Job drawing, mm, ordinate dimensions from the low corner. One solid piece. A direction names the side the tool comes from. Round coordinates to 2 decimals unless told otherwise and drop trailing zeros. Loops run counter-clockwise (first coordinate to the right, second up) from the corner with the lowest first, then second, coordinate; pieces in that order, holes last.
1) 3-axis set-ups, long thin cutter, end or side, ignore diameter. For the marked faces 1 and 2: which of +Z, -Z, +X, -X, +Y, -Y reach the whole face in a straight line?
2) Band-saw the part on B-B, the plane x = 48.5. Write the cut outline in (y, z).
3) Mould opens along Z. For the marked faces 3, 4 and 5 say: +Z half, -Z half, draft (parallel to the pull), parting line (faces both ways), or undercut.
4) Probe line 1 (X direction, y = 16, z = 61); line 2 (Z direction, x = 138.5, y = 27). List the from-to ranges inside material, lowest first.
5) Drop a flat-ended pin along its axis: P1, Ø10, axis at x = 246.5, y = 14.5, coming from the -Z side. Give the stop position or say it passes through.
6) Band-saw the part on C-C, the plane z = 81.5. Write the cut outline in (x, y).
7) Band-saw the part on A-A, the plane y = 23. Write the cut outline in (x, z), then the cut area to 3 significant figures.
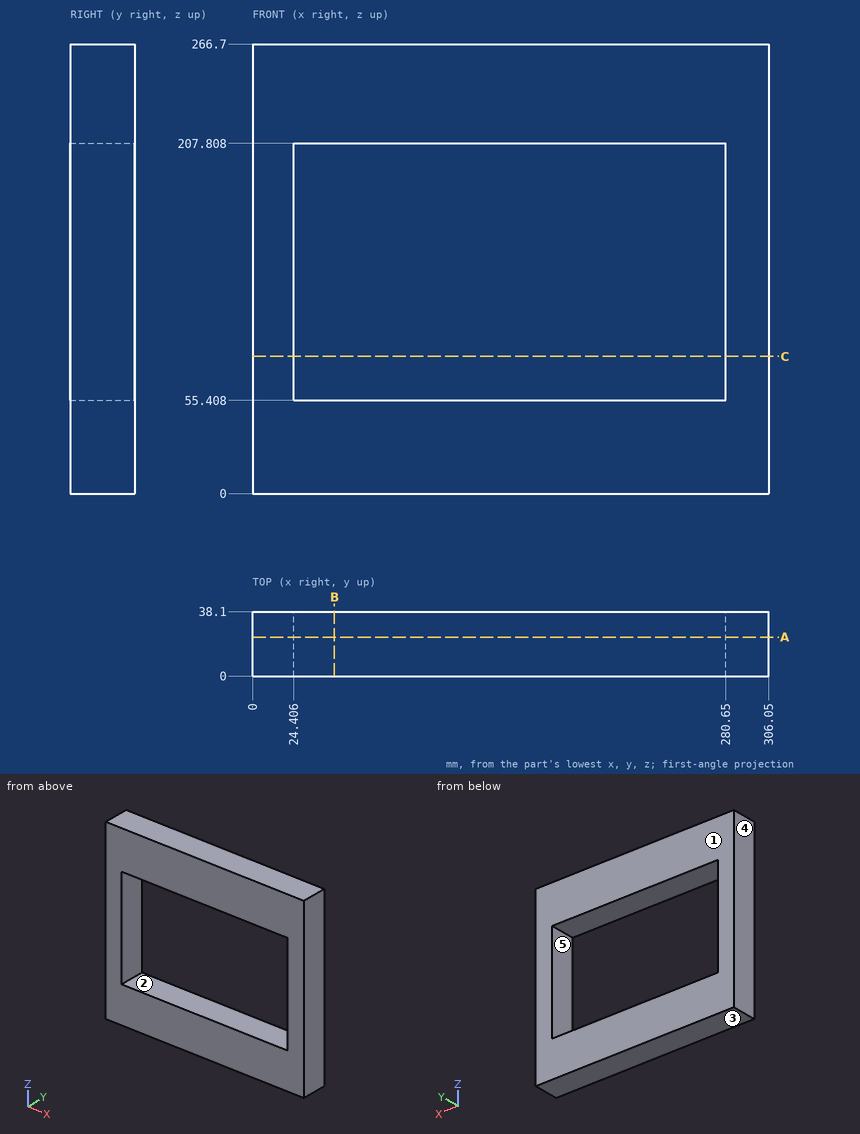
Reported:
1. face 1: +Z, -Z, +X, -X, +Y
1. face 2: +Y, -Y
2. outline: (0, 0) - (38.1, 0) - (38.1, 55.41) - (0, 55.41) - close; (0, 207.81) - (38.1, 207.81) - (38.1, 266.7) - (0, 266.7) - close
3. face 3: -Z half
3. face 4: draft
3. face 5: undercut
4. line 1: x = 0 to 24.41, 280.65 to 306.05
4. line 2: z = 0 to 55.41, 207.81 to 266.7
5. P1: stops at z = 0
6. outline: (0, 0) - (24.41, 0) - (24.41, 38.1) - (0, 38.1) - close; (280.65, 0) - (306.05, 0) - (306.05, 38.1) - (280.65, 38.1) - close
7. outline: (0, 0) - (306.05, 0) - (306.05, 266.7) - (0, 266.7) - close; hole (24.41, 55.41) - (280.65, 55.41) - (280.65, 207.81) - (24.41, 207.81) - close
7. area: 42,600 mm2
